```python
from build123d import *

# Parameters (mm, degrees)
F0_W     = 160
F0_H     = 320
F0_R     = 3
F0_R_2   = 17.5
F1_DEPTH = 2.5


# Not quite as in the source:
# - a fillet or chamfer that OpenCascade refuses, or shapes differently, is made with other operations: its cross-section is extruded or revolved along the edge and cut away or added


with BuildPart() as f1:
    # F0 (on Front) → F1 (new body)
    with BuildSketch(Plane.XZ):
        with Locations((-1.8876045942, 29.6809725389)):
            Rectangle(F0_W, F0_H)
        with Locations((-1.8876045942, -95.3190274611)):
            Circle(F0_R, mode=Mode.SUBTRACT)
        with Locations((-1.8876045942, -10.3190274611)):
            Circle(F0_R_2, mode=Mode.SUBTRACT)
        with Locations((-1.8876045942, 154.6809725389)):
            Circle(F0_R, mode=Mode.SUBTRACT)
    extrude(amount=F1_DEPTH)

    # F2: chamfer of 4 on 2 edges, made by hand

    # F2_s1 → F2_t2 (revolve, cut)
    with BuildSketch(Plane.XY.offset(154.6809725389)):
        Polygon((1.1123954058, 1.5), (5.1123954058, -2.5), (1.1123954058, -2.5), align=None)
    revolve(axis=Axis((-1.8876045942, -2.5, 154.6809725389), (0, -1, 0)), mode=Mode.SUBTRACT)

    # F2_s3 → F2_t4 (revolve, cut)
    with BuildSketch(Plane.XY.offset(-95.3190274611)):
        Polygon((1.1123954058, 1.5), (5.1123954058, -2.5), (1.1123954058, -2.5), align=None)
    revolve(axis=Axis((-1.8876045942, -2.5, -95.3190274611), (0, -1, 0)), mode=Mode.SUBTRACT)


solid = f1.part
```
Build history of the part. All positions in model axes, mm. Coordinates: 2 decimals unless noted, no trailing zeros. Order: outer loops, then holes, each group sorted by start corner. A loop starts at its lowest first (then second) coordinate and runs counter-clockwise, first axis right, second up. Notation, with made-up numbers: (31.5, 67.5) -> (87.5, 67.5) arc R12 cw to (87.5, 87.5) -> close; hole circle Ø9 at (19.5, -35.5). An arc over 180 degrees is marked (long way). Answer in a Markdown table with one row per item. Add a question column.
Q1. Band-saw the part on B-B, the plane y = -1.4. List the corners of the cut face in (x, z), then the cut area to 3 significant figures.
Q2. Mould opens along Z. For faces 1 (the face through (0.62, -0.16, 158.61)), 2 (the face through (14.804, -1.232, -5.063)), 3 (the face through (-3, -2.5, 32)) say: +Z half, -Z half, draft (parallel to the pull), parting line (faces both ways), or undercut.
Q3. Band-saw the part on A-A, the plane x = -13. List the corners of the cut face in (y, z).
Q4. Wall check: line 1 along Z through (x, y) = (9.5, -0.35); line 2 along X through (y, z) = (-0.4, -23.5); line 3 along X through (y, z) = (-0.75, -100). Give the ranges that are in metal, low to high. Write a range as [from, to].
Answers follow:
| question | item | result |
|---|---|---|
| 1 | outline | (-81.89, -130.32) -> (78.11, -130.32) -> (78.11, 189.68) -> (-81.89, 189.68) -> close; hole circle Ø35 at (-1.89, -10.32); hole circle Ø11.8 at (-1.89, -95.32); hole circle Ø11.8 at (-1.89, 154.68) |
| 1 | area | 50,000 mm^2 |
| 2 | face 1 | undercut |
| 2 | face 2 | undercut |
| 2 | face 3 | draft |
| 3 | outline | (-2.5, -130.32) -> (0, -130.32) -> (0, -23.84) -> (-2.5, -23.84) -> close; (-2.5, 3.2) -> (0, 3.2) -> (0, 189.68) -> (-2.5, 189.68) -> close |
| 4 | line 1 | [-130.32, -23.61], [2.97, 189.68] |
| 4 | line 2 | [-81.89, -13.4], [9.62, 78.11] |
| 4 | line 3 | [-81.89, -4.26], [0.49, 78.11] |
